The listing builds one solid part. Answer for the finished solid, in the listing's coordinates (mm). Face numbers are marked on the shaded views. A direction names the side the tool comes from. Coordinates: 2 decimals unless noted, no trailing zeros. Order: outer loops, then holes, each group sorted by start corner. A loop starts at its lowest first (then second) coordinate and runs counter-clockwise, first axis right, second up. Notation, with made-up numbers: (6.25, 45.5) - (40.25, 45.5) arc R26 cw to (40.25, 60.5) - close; hole circle Ø9 at (24.25, -26). An arc over 180 degrees is marked (long way). Use a Markdown table: item, result. Add a question column.
Item 1: Find the intervals of material crossed by line 1 along Y through (x, z) = (30.5, 21); line 2 along X through (y, z) = (13, -8); line 3 along Y through (x, z) = (-12, 23.5), in increasing order.
Item 2: The part is cut by section A-A, the plane y = 15. Give the vertices of the cut face in (x, z).
Item 3: The part is cut by section C-C, the plane x = 8. Give the vertices of the cut face in (y, z), then the cut area to 3 significant figures.
Item 4: The part is cut by section D-D, the plane y = 24. Give the vertices of the cut face in (x, z), then the cut area to 3 significant figures.
Item 5: Flat-ended cylindrical pins translate along their axes: P1, Ø1.5, axis at x = -25, z = 23.5, coming from the -Y side; P2, Ø6, axis at y = -1, z = -7.5, coming from the -X side; P3, Ø3.5, axis at x = 33.5, y = -4, coming from the -Z side; P4, Ø1, axis at x = 3.5, z = -6, coming from the +Y side. Find the tip coordinate at first contact, or state that the pin passes through.
Item 6: The part is cut by section B-B, the plane z = 13. Give the vertices of the cut face in (x, y), then the cut area to 3 significant figures.
Item 7: The mould has two halves that part along X. Classify the marked faces 1, 2 and 3: released by +X, released by -X, zero draft, split by the parting line, or undercut.
Item 8: For the marked faces 4, 5, 6 and 7, determine the directions among +Z, -Z, +X, -X, +Y, -Y from which every point of the face is accessible in a straight line to the end or side of a thin tool.
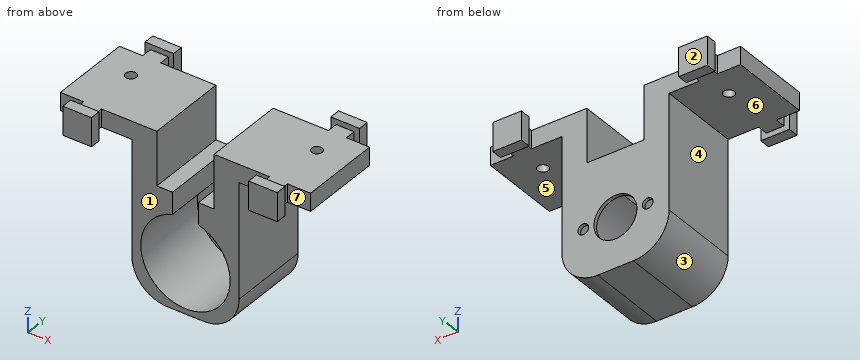
Autodesk Inventor part; units mm, degrees
ref_plane "YZ Plane" through (0, 0, 0) normal (1, 0, 0) x (0, 1, 0)
ref_plane "XZ Plane" through (0, 0, 0) normal (0, 1, 0) x (-1, 0, 0)
ref_plane "XY Plane" through (0, 0, 0) normal (0, 0, 1) x (1, 0, 0)
sketch "Esquisse1" plane through (0, 0, 0) normal (0, 1, 0) x (-1, 0, 0)
  line L0 (7.2872, 10.2128) -> (-22.7128, 10.2128)
  line L1 (-22.7128, 10.2128) -> (-22.7128, -19.7872)
  line L2 (-22.7128, -19.7872) -> (7.2872, -19.7872)
  line L3 (7.2872, -19.7872) -> (7.2872, 10.2128)
  point P0 (0, 0)
  dimension "d0" = 30
  dimension "d1" = 30
extrude "Extrusion1" add sketch "Esquisse1" along normal blind 23
ref_plane "Plan médian" through (7.7128, 0, 10.2128) normal (1, 0, 0) x (0, 0, -1)
sketch "Esquisse4" plane through (0, 0, 0) normal (0, -1, 0) x (1, 0, 0)
  circle A0 centre (7.7128, -7.8122) radius 11.975
  line L0 (-7.2872, 10.2128) -> (22.7128, 10.2128)
  line L1 (4.1002, 3.6049) -> (4.1002, 10.2128)
  line L2 (11.3254, 3.6049) -> (11.3254, 10.2128)
  point P0 (0, 0)
extrude "Extrusion2" cut sketch "Esquisse4" against normal blind 22
sketch "Esquisse5" plane through (0, 22, 0) normal (0, -1, 0) x (1, 0, 0)
  circle A0 centre (7.7128, -7.8122) radius 6
  circle A1 centre (16.7128, -7.5941) radius 1.5
  circle A2 centre (-1.2872, -7.5941) radius 1.5
  point P0 (0, 0)
  dimension "d66" = 3
  dimension "d67" = 3
  dimension "d68" = 9
  dimension "d69" = 9
extrude "Extrusion3" cut sketch "Esquisse5" against normal through all
sketch "Esquisse6" plane through (-7.2872, 23, 10.2128) normal (0, 0, 1) x (1, 0, 0)
  line L0 (0, -23) -> (11.3874, -23)
  line L1 (5.9558, 0) -> (8.4558, 0)
  line L2 (0, -23) -> (7, -23)
  line L3 (7, -23) -> (7, 0)
  line L4 (7, 0) -> (0, 0)
  line L5 (0, 0) -> (0, -23)
  line L6 (30, -23) -> (30, 0)
  line L7 (0, 0) -> (30, 0)
  line L8 (30, -23) -> (23, -23)
  line L9 (23, -23) -> (23, 0)
  line L10 (23, 0) -> (30, 0)
  line L11 (30, 0) -> (30, -23)
  point P0 (7.2872, -23)
  point P1 (12, -23)
  point P2 (11.5355, -23)
  dimension "d8" = 7
  dimension "d9" = 7
extrude "Extrusion4" add sketch "Esquisse6" along normal blind 10
sketch "Esquisse7" plane through (-7.2872, 23, 20.2128) normal (0, 0, 1) x (1, 0, 0)
  line L0 (7, 0) -> (-20, 0)
  line L1 (-20, 0) -> (-20, -23)
  line L2 (-20, -23) -> (7, -23)
  line L3 (7, -23) -> (7, 0)
  line L4 (30, 0) -> (0, 0)
  line L5 (23, 0) -> (50, 0)
  line L6 (50, 0) -> (50, -23)
  line L7 (50, -23) -> (23, -23)
  line L8 (23, -23) -> (23, 0)
  line L9 (0, 0) -> (0, -23)
  line L10 (30, -23) -> (30, 0)
  point P0 (7.2872, -23)
  dimension "d12" = 20
  dimension "d13" = 20
extrude "Extrusion5" add sketch "Esquisse7" along normal blind 5
sketch "Esquisse8" plane through (0, 23, 0) normal (0, 1, 0) x (1, 0, 0)
  line L0 (36.2128, -25.2128) -> (31.2128, -25.2128)
  line L1 (31.2128, -25.2128) -> (31.2128, -20.2128)
  line L2 (31.2128, -20.2128) -> (36.2128, -20.2128)
  line L3 (36.2128, -20.2128) -> (36.2128, -25.2128)
  line L4 (42.7128, -20.2128) -> (42.7128, -25.2128)
  line L5 (42.7128, -20.2128) -> (22.7128, -20.2128)
  line L6 (-0.2872, -25.2128) -> (-27.2872, -25.2128)
  line L7 (-27.2872, -20.2128) -> (-27.2872, -25.2128)
  line L8 (-20.7872, -25.2128) -> (-15.7872, -25.2128)
  line L9 (-15.7872, -25.2128) -> (-15.7872, -20.2128)
  line L10 (-15.7872, -20.2128) -> (-20.7872, -20.2128)
  line L11 (-20.7872, -20.2128) -> (-20.7872, -25.2128)
  line L12 (-7.2872, -20.2128) -> (-27.2872, -20.2128)
  point P0 (0, 0)
  point P1 (-0.4939, -25.2128)
  dimension "d16" = 6.5
  dimension "d17" = 5
  dimension "d18" = 5
  dimension "d19" = 0
  dimension "d53" = 5
  dimension "d54" = 5
  dimension "d55" = 0
  dimension "d57" = 6.5
extrude "Extrusion6" add sketch "Esquisse8" along normal blind 3 contours L0 L1 L2 L3 | L6 L11 L10 L9
sketch "Esquisse9" plane through (0, 26, 0) normal (0, 1, 0) x (1, 0, 0)
  line L0 (37.7128, -26.7128) -> (29.7128, -26.7128)
  line L1 (29.7128, -26.7128) -> (29.7128, -18.7128)
  line L2 (29.7128, -18.7128) -> (37.7128, -18.7128)
  line L3 (37.7128, -18.7128) -> (37.7128, -26.7128)
  line L4 (42.7128, -20.2128) -> (42.7128, -25.2128)
  line L5 (-27.2872, -25.2128) -> (-0.2872, -25.2128)
  line L6 (-27.2872, -20.2128) -> (-27.2872, -25.2128)
  line L7 (31.2128, -25.2128) -> (15.7128, -25.2128)
  line L8 (-14.2872, -26.7128) -> (-22.2872, -26.7128)
  line L9 (-22.2872, -26.7128) -> (-22.2872, -18.7128)
  line L10 (-22.2872, -18.7128) -> (-14.2872, -18.7128)
  line L11 (-14.2872, -18.7128) -> (-14.2872, -26.7128)
  point P0 (0, 0)
  point P1 (-13.7872, -25.2128)
  dimension "d25" = 8
  dimension "d26" = 5
  dimension "d59" = 8
  dimension "d60" = 1.5
  dimension "d62" = 5
  dimension "d63" = 1.5
  dimension "d64" = 8
  dimension "d65" = 8
extrude "Extrusion7" add sketch "Esquisse9" along normal blind 3
sketch "Esquisse10" plane through (22.7128, 23, -19.7872) normal (0, 0, -1) x (-1, 0, 0)
  line L0 (0, -23) -> (15, -23)
  line L1 (15, -23) -> (15, -1)
  line L2 (15, -23) -> (30, -23)
  line L3 (30, -23) -> (30, 0)
  line L4 (0, 0) -> (30, 0)
  line L5 (0, -23) -> (0, 0)
  line L6 (0, 0) -> (30, 0)
  line L7 (30, 0) -> (30, -23)
  line L8 (30, -23) -> (0, -23)
  line L9 (0, -23) -> (0, 0)
  point P0 (22.7128, -23)
extrude "Extrusion8" add sketch "Esquisse10" along normal blind 2
fillet "Congé1" radius 10 2 edges at (22.7128, 11.5, -21.7872) (-7.2872, 11.5, -21.7872)
sketch "Esquisse12" plane through (0, 0, 0) normal (0, -1, 0) x (1, 0, 0)
  arc A0 (4.1002, 3.6049) -> (11.3254, 3.6049) centre (7.7128, -7.8122) ccw
  circle A1 centre (7.7128, -7.8122) radius 12.5
  point P0 (0, 0)
  dimension "d42" = 25
extrude "Extrusion10" cut sketch "Esquisse12" against normal up to surface (22 mm away)
sketch "Esquisse13" plane through (-7.2872, 23, 25.2128) normal (0, 0, 1) x (1, 0, 0)
  circle A0 centre (-11, -8) radius 1.5
  circle A1 centre (41, -8) radius 1.5
  line L0 (7, 0) -> (-20, 0)
  line L1 (-20, 0) -> (-20, -23)
  line L2 (50, 0) -> (23, 0)
  line L3 (50, -23) -> (50, 0)
  point P0 (7.2872, -23)
  dimension "d45" = 3
  dimension "d46" = 3
  dimension "d49" = 8
  dimension "d50" = 9
  dimension "d51" = 8
  dimension "d52" = 9
extrude "Extrusion11" cut sketch "Esquisse13" against normal through all
sketch "Esquisse14" plane through (0, 0, 0) normal (0, -1, 0) x (1, 0, 0)
  line L0 (-27.2872, 20.2128) -> (-7.2872, 20.2128)
  line L1 (-27.2872, 25.2128) -> (-0.2872, 25.2128)
  line L2 (-20.7872, 20.2128) -> (-15.7872, 20.2128)
  line L3 (-15.7872, 20.2128) -> (-15.7872, 25.2128)
  line L4 (-15.7872, 25.2128) -> (-20.7872, 25.2128)
  line L5 (-20.7872, 25.2128) -> (-20.7872, 20.2128)
  line L6 (-27.2872, 20.2128) -> (-27.2872, 25.2128)
  line L7 (15.7128, 25.2128) -> (42.7128, 25.2128)
  line L8 (31.2128, 20.2128) -> (36.2128, 20.2128)
  line L9 (36.2128, 20.2128) -> (36.2128, 25.2128)
  line L10 (36.2128, 25.2128) -> (31.2128, 25.2128)
  line L11 (31.2128, 25.2128) -> (31.2128, 20.2128)
  line L12 (42.7128, 20.2128) -> (42.7128, 25.2128)
  point P0 (0, 0)
  dimension "d70" = 6.5
  dimension "d71" = 5
  dimension "d72" = 6.5
  dimension "d73" = 5
  dimension "d74" = 5
extrude "Extrusion12" add sketch "Esquisse14" along normal blind 3 contours L5 L1 L3 L0 | L7 L9 L8 L11
sketch "Esquisse17" plane through (0, -3, 0) normal (0, -1, 0) x (1, 0, 0)
  line L0 (37.7128, 18.7128) -> (29.7128, 18.7128)
  line L1 (29.7128, 18.7128) -> (29.7128, 26.7128)
  line L2 (29.7128, 26.7128) -> (37.7128, 26.7128)
  line L3 (37.7128, 26.7128) -> (37.7128, 18.7128)
  line L4 (-14.2872, 18.7128) -> (-22.2872, 18.7128)
  line L5 (-22.2872, 18.7128) -> (-22.2872, 26.7128)
  line L6 (-22.2872, 26.7128) -> (-14.2872, 26.7128)
  line L7 (-14.2872, 26.7128) -> (-14.2872, 18.7128)
  line L8 (-27.2872, 20.2128) -> (-27.2872, 25.2128)
  line L9 (-20.7872, 20.2128) -> (-15.7872, 20.2128)
  line L10 (42.7128, 20.2128) -> (42.7128, 25.2128)
  line L11 (31.2128, 20.2128) -> (36.2128, 20.2128)
  point P0 (0, 0)
  dimension "d86" = 5
  dimension "d87" = 8
  dimension "d88" = 8
  dimension "d89" = 1.5
  dimension "d90" = 5
  dimension "d91" = 8
  dimension "d92" = 8
  dimension "d93" = 1.5
extrude "Extrusion14" add sketch "Esquisse17" along normal blind 3
properties part number "support_codeur"
Solution:
| question | item | result |
|---|---|---|
| 1 | line 1 | y = -6 to -3, 0 to 23, 26 to 29 |
| 1 | line 2 | x = -7.29 to -4.79, 20.21 to 22.71 |
| 1 | line 3 | y = 0 to 23 |
| 2 | outline | (-27.29, 20.21) - (-19.79, 20.21) - (-19.79, 25.21) - (-27.29, 25.21) - close; (-16.79, 20.21) - (-7.29, 20.21) - (-7.29, -11.79) arc R10 ccw to (2.71, -21.79) - (12.71, -21.79) arc R10 ccw to (22.71, -11.79) - (22.71, 20.21) - (32.21, 20.21) - (32.21, 25.21) - (15.71, 25.21) - (15.71, 10.21) - (11.33, 10.21) - (11.33, 4.15) arc R12.5 cw (long way) to (4.1, 4.15) - (4.1, 10.21) - (-0.29, 10.21) - (-0.29, 25.21) - (-16.79, 25.21) - close; (35.21, 20.21) - (42.71, 20.21) - (42.71, 25.21) - (35.21, 25.21) - close |
| 3 | outline | (0, -21.79) - (23, -21.79) - (23, -13.81) - (22, -13.81) - (22, -20.31) - (0, -20.31) - close; (22, -1.82) - (23, -1.82) - (23, 10.21) - (22, 10.21) - close |
| 3 | area | 52.5 mm2 |
| 4 | outline | (-20.79, 20.21) - (-15.79, 20.21) - (-15.79, 25.21) - (-20.79, 25.21) - close; (31.21, 20.21) - (36.21, 20.21) - (36.21, 25.21) - (31.21, 25.21) - close |
| 4 | area | 50.0 mm2 |
| 5 | P1 | stops at y = 0 |
| 5 | P2 | stops at x = -7.29 |
| 5 | P3 | stops at z = 18.71 |
| 5 | P4 | passes through |
| 6 | outline | (-7.29, 0) - (-0.29, 0) - (-0.29, 23) - (-7.29, 23) - close; (15.71, 0) - (22.71, 0) - (22.71, 23) - (15.71, 23) - close |
| 6 | area | 322 mm2 |
| 7 | face 1 | undercut |
| 7 | face 2 | zero draft |
| 7 | face 3 | released by -X |
| 8 | face 4 | -Z, -X, +Y, -Y |
| 8 | face 5 | -Z, +X |
| 8 | face 6 | -Z, -X |
| 8 | face 7 | +Z, -Z, +X |
